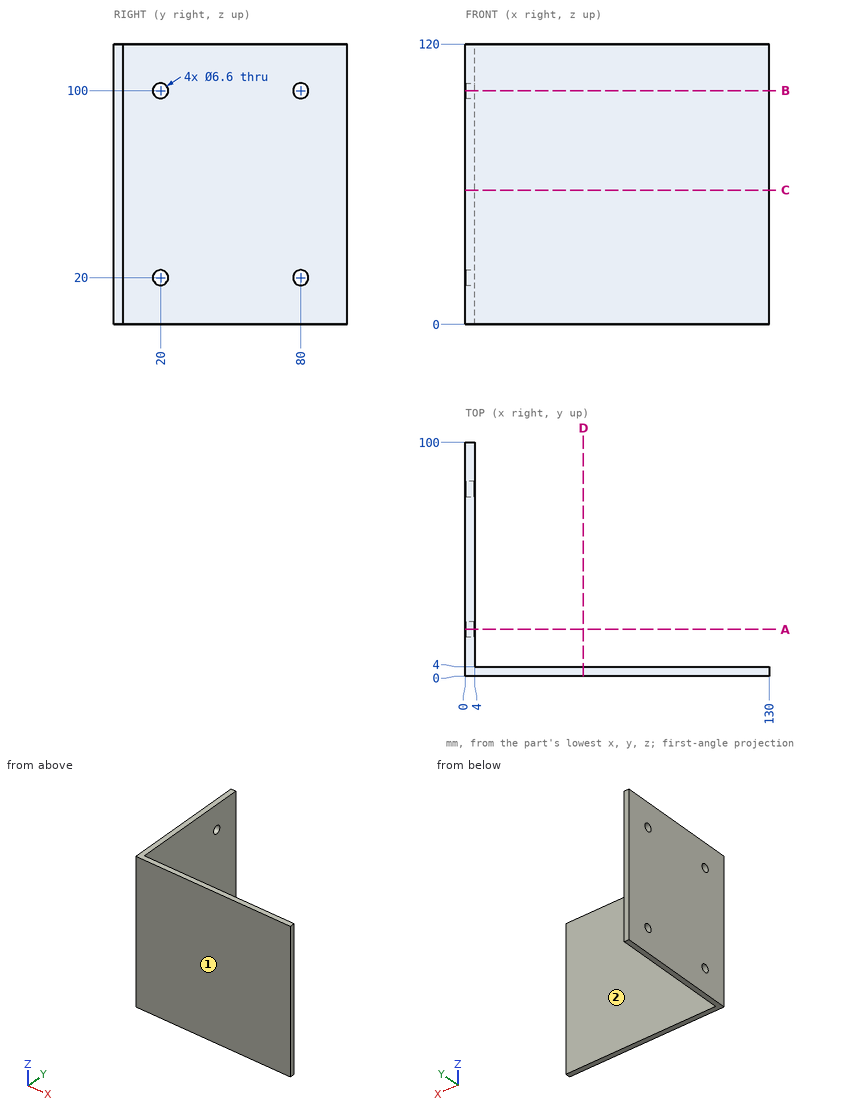
Verification items for this drawing (mm, ordinates from the low corner). A direction names the side the tool comes from. Coordinates: 2 decimals unless noted, no trailing zeros. Write each loop counter-clockwise with the first axis right and the second up, starting at its lowest first coordinate (ties: lowest second). Pieces come first, ordered by that corner, then holes. Notation, with made-up numbers: M 28,-38 L 87,-38 A9 ccw 87,-27 Z; hole C 29.25,89.5 d4. An arc over 180 degrees is marked long. Use one line per item in the form item = value. Start each with the question number.
1) Thickness scan on probe 1 along Z at (x, y) = (1.7, 20); probe 2 along X at (y, z) = (58.5, 64). Record the ranges inside material, lowest first. Write a range as from..to.
2) Go/stop test with flat-tipped pins: pin 1 Ø10.5 at (y, z) = (20, 20) entering from +X; pin 2 Ø4 at (y, z) = (20, 100) entering from -X. Record where each tip stops, or that it passes through.
3) Section check C-C on z = 57.5. Enter the section's corners in (x, y).
4) Section check B-B on z = 100. Enter the section's corners in (x, y).
5) Section check D-D on x = 50.5. Enter the section's corners in (y, z), and give its area (3 significant figures).
6) Set-up check for the marked faces 1 and 2: record each of +Z, -Z, +X, -X, +Y, -Y from which the full face is reachable in a straight line by a thin tool's end or side.
7) Section check A-A on y = 20. Enter the section's corners in (x, z), and give its area (3 significant figures).
Responses:
q1.probe_1 = 0..16.7, 23.3..96.7, 103.3..120
q1.probe_2 = 0..4
q2.pin_1 = 4
q2.pin_2 = through
q3.outline = M 0,0 L 130,0 L 130,4 L 4,4 L 4,100 L 0,100 Z
q4.outline = M 0,0 L 130,0 L 130,4 L 4,4 L 4,16.7 L 0,16.7 Z; M 0,23.3 L 4,23.3 L 4,76.7 L 0,76.7 Z; M 0,83.3 L 4,83.3 L 4,100 L 0,100 Z
q5.outline = M 0,0 L 4,0 L 4,120 L 0,120 Z
q5.area = 480 mm2
q6.face_1 = +Z, -Z, +X, -X, -Y
q6.face_2 = +Z, -Z, +X, +Y
q7.outline = M 0,0 L 4,0 L 4,16.7 L 0,16.7 Z; M 0,23.3 L 4,23.3 L 4,96.7 L 0,96.7 Z; M 0,103.3 L 4,103.3 L 4,120 L 0,120 Z
q7.area = 427 mm2
